Part model, mm, in its own coordinate system. Face numbers are marked on the shaded views. Coordinates: 2 decimals unless noted, no trailing zeros. Order: outer loops, then holes, each group sorted by start corner. A loop starts at its lowest first (then second) coordinate and runs counter-clockwise, first axis right, second up.
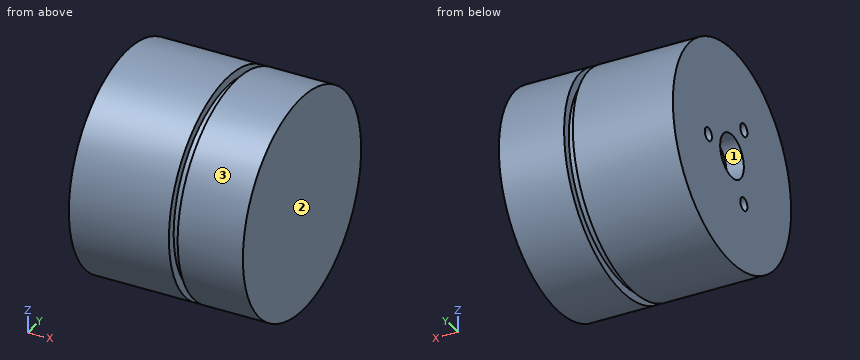
from build123d import *

# Parameters (mm, degrees)
SKETCH_1_R          = 2.5
EXTRUDE_1_DEPTH     = 2.5
SKETCH_3_R          = 2.4
EXTRUDE_4_DEPTH     = 1.5
CUT_EXTRUDE_START   = -0.2
SKETCH_4_R          = 2.5
SKETCH_4_R_2        = 2.3
CUT_EXTRUDE_2_DEPTH = 0.2
SKETCH_5_R          = 2.5
SKETCH_5_R_2        = 2.4
EXTRUDE_5_DEPTH     = 1.5
SKETCH_6_R          = 0.5
CUT_EXTRUDE_3_DEPTH = 0.4
SKETCH_7_R          = 0.15
CUT_EXTRUDE_4_DEPTH = 0.8


with BuildPart() as part:
    # 草图1 → 凸台-拉伸1 (new body)
    with BuildSketch(Plane(origin=(0, 0, 0), x_dir=(0, 0, -1), z_dir=(1, 0, 0))):
        Circle(SKETCH_1_R)
    extrude(amount=EXTRUDE_1_DEPTH)

    # 草图3 → 凸台-拉伸4 (add)
    with BuildSketch(Plane(origin=(2.5, 0, 0), x_dir=(0, 0, -1), z_dir=(1, 0, 0))):
        Circle(SKETCH_3_R)
    extrude(amount=EXTRUDE_4_DEPTH)

    # 草图4 → 切除-拉伸2 (cut)
    with BuildSketch(Plane(origin=(2.5, 0, 0), x_dir=(0, 0, -1), z_dir=(1, 0, 0)).offset(CUT_EXTRUDE_START)):
        Circle(SKETCH_4_R)
        Circle(SKETCH_4_R_2, mode=Mode.SUBTRACT)
    extrude(amount=CUT_EXTRUDE_2_DEPTH, mode=Mode.SUBTRACT)

    # 草图5 → 凸台-拉伸5 (add)
    with BuildSketch(Plane.ZY.offset(-2.5)):
        with Locations(Location((0, 0, 0), (0, 0, 180))):
            Circle(SKETCH_5_R)
        Circle(SKETCH_5_R_2, mode=Mode.SUBTRACT)
    extrude(amount=-EXTRUDE_5_DEPTH)

    # 草图6 → 切除-拉伸3 (cut)
    with BuildSketch(Plane.ZY):
        Circle(SKETCH_6_R)
    extrude(amount=-CUT_EXTRUDE_3_DEPTH, mode=Mode.SUBTRACT)

    # 草图7 → 切除-拉伸4 (cut)
    with BuildSketch(Plane.ZY):
        with Locations((0, 1)):
            Circle(SKETCH_7_R)
        with Locations((-0.866025404, -0.5)):
            Circle(SKETCH_7_R)
        with Locations((0.866025404, -0.5)):
            Circle(SKETCH_7_R)
    extrude(amount=-CUT_EXTRUDE_4_DEPTH, mode=Mode.SUBTRACT)


solid = part.part
Q1. Wall check: line 1 along X through (y, z) = (2.2, -0.85); line 2 along Z through (x, y) = (1.75, 0.1); line 3 along X through (y, z) = (0.35, 0.05). Give the ranges that are in metal, low to high.
Results list:
line 1: x = 0 to 2.3, 2.5 to 4
line 2: z = -2.5 to 2.5
line 3: x = 0.4 to 4
Q2. Cut at B-B on y = -0.85. Write the cut outline in (x, z).
Results list:
outline: (0, -2.35) - (2.3, -2.35) - (2.3, -2.14) - (2.5, -2.14) - (2.5, -2.35) - (4, -2.35) - (4, 2.35) - (2.5, 2.35) - (2.5, 2.14) - (2.3, 2.14) - (2.3, 2.35) - (0, 2.35) - close
Q3. Mould opens along Z. For the marked faces 1, 2 and 3 say: pulls with the +Z half, pulls with the -Z half, needs draft (parallel to the pull), parting line crosses it, or undercut.
Results list:
face 1: undercut
face 2: needs draft
face 3: parting line crosses it
Q4. Cut at A-A on z = 0. Write the cut outline in (x, y).
Results list:
outline: (0, -2.5) - (2.3, -2.5) - (2.3, -2.3) - (2.5, -2.3) - (2.5, -2.5) - (4, -2.5) - (4, 2.5) - (2.5, 2.5) - (2.5, 2.3) - (2.3, 2.3) - (2.3, 2.5) - (0, 2.5) - (0, 1.15) - (0.8, 1.15) - (0.8, 0.85) - (0, 0.85) - (0, 0.5) - (0.4, 0.5) - (0.4, -0.5) - (0, -0.5) - close
Q5. Cut at D-D on z = 0.9. Write the cut outline in (x, y), and give its area (3 significant figures).
Results list:
outline: (0, -2.33) - (2.3, -2.33) - (2.3, -2.12) - (2.5, -2.12) - (2.5, -2.33) - (4, -2.33) - (4, 2.33) - (2.5, 2.33) - (2.5, 2.12) - (2.3, 2.12) - (2.3, 2.33) - (0, 2.33) - (0, -0.35) - (0.8, -0.35) - (0.8, -0.65) - (0, -0.65) - close
area: 18.3 mm2
Q6. Cut at C-C on x = 1.15. Write the cut outline in (y, z), and give its area (3 significant figures).
Results list:
outline: circle Ø5 at (0, 0)
area: 19.6 mm2
